```python
from build123d import *

# Parameters (mm, degrees)
SKETCH_1_W          = 55
SKETCH_1_H          = 60
EXTRUDE_1_DEPTH     = 3
SKETCH_2_W          = 30
SKETCH_2_H          = 22
EXTRUDE_2_DEPTH     = 3
SKETCH_3_R          = 1.05
CUT_EXTRUDE_1_DEPTH = 3
SKETCH_4_R          = 1.525
CUT_EXTRUDE_2_DEPTH = 3
SKETCH_5_R          = 1.5
CUT_EXTRUDE_3_DEPTH = 10
SKETCH_6_R          = 1.5
CUT_EXTRUDE_4_DEPTH = 10
CUT_EXTRUDE_5_DEPTH = 10
FILLET_1_R          = 2
FILLET_2_R          = 2


with BuildPart() as part:
    # 草图1 → 凸台-拉伸1 (new body)
    with BuildSketch(Plane.XY):
        Rectangle(SKETCH_1_W, SKETCH_1_H)
    extrude(amount=EXTRUDE_1_DEPTH)

    # 草图2 → 凸台-拉伸2 (add)
    with BuildSketch(Plane(origin=(0, 0, 0), x_dir=(-1, 0, 0), z_dir=(0, 0, -1))):
        with Locations((0, 30)):
            Rectangle(SKETCH_2_W, SKETCH_2_H)
    extrude(amount=-EXTRUDE_2_DEPTH)

    # 草图3 → 切除-拉伸1 (cut)
    with BuildSketch(Plane(origin=(0, 0, 0), x_dir=(-1, 0, 0), z_dir=(0, 0, -1))):
        with Locations((-16.05, 30)):
            Circle(SKETCH_3_R)
        with Locations((16.05, 30)):
            Circle(SKETCH_3_R)
    extrude(amount=-CUT_EXTRUDE_1_DEPTH, mode=Mode.SUBTRACT)

    # 草图4 → 切除-拉伸2 (cut)
    with BuildSketch(Plane.XY.offset(3)):
        with Locations((-10, 38)):
            Circle(SKETCH_4_R)
        with Locations((10, 38)):
            Circle(SKETCH_4_R)
    extrude(amount=-CUT_EXTRUDE_2_DEPTH, mode=Mode.SUBTRACT)

    # 草图5 → 切除-拉伸3 (cut)
    with BuildSketch(Plane(origin=(0, 0, 0), x_dir=(-1, 0, 0), z_dir=(0, 0, -1))):
        with Locations((-18.5, -17.5)):
            Circle(SKETCH_5_R)
        with Locations((18.5, -17.5)):
            Circle(SKETCH_5_R)
    extrude(amount=-CUT_EXTRUDE_3_DEPTH, mode=Mode.SUBTRACT)

    # 草图6 → 切除-拉伸4 (cut)
    with BuildSketch(Plane.XY.offset(3)):
        with Locations((20, 15)):
            Circle(SKETCH_6_R)
        with Locations((-20, 15)):
            Circle(SKETCH_6_R)
    extrude(amount=-CUT_EXTRUDE_4_DEPTH, mode=Mode.SUBTRACT)

    # 草图7 → 切除-拉伸5 (cut)
    with BuildSketch(Plane.XY.offset(3)):
        Polygon((-15, 24), (15, 24), (15, -12.5), (13.5, -12.5), (13.5, -24), (-13.5, -24), (-13.5, -12.5), (-15, -12.5), align=None)
    extrude(amount=-CUT_EXTRUDE_5_DEPTH, mode=Mode.SUBTRACT)

    # 圆角1
    # the kernel refuses this fillet: 2 mm, written as the material it adds along each edge
    with BuildSketch(Plane(origin=(-15, 24, 3), x_dir=(0, -1, 0), z_dir=(0, 0, -1))) as fillet_1_piece_1:
        with BuildLine():
            CenterArc((FILLET_1_R, -FILLET_1_R), FILLET_1_R, 90, 90)
            Line((0, -FILLET_1_R), (-FILLET_1_R * 0.02, -FILLET_1_R))
            Line((-FILLET_1_R * 0.02, -FILLET_1_R), (-FILLET_1_R * 0.02, FILLET_1_R * 0.02))
            Line((-FILLET_1_R * 0.02, FILLET_1_R * 0.02), (FILLET_1_R, FILLET_1_R * 0.02))
            Line((FILLET_1_R, FILLET_1_R * 0.02), (FILLET_1_R, 0))
        make_face()
    extrude(amount=3)
    with BuildSketch(Plane(origin=(15, 24, 3), x_dir=(0, -1, 0), z_dir=(0, 0, -1)), Plane(origin=(-13.5, -24, 3), x_dir=(0, 1, 0), z_dir=(0, 0, -1)), Plane(origin=(13.5, -24, 3), x_dir=(-1, 0, 0), z_dir=(0, 0, -1))) as fillet_1_piece_2:
        with BuildLine():
            CenterArc((FILLET_1_R, FILLET_1_R), FILLET_1_R, 180, 90)
            Line((0, FILLET_1_R), (-FILLET_1_R * 0.02, FILLET_1_R))
            Line((-FILLET_1_R * 0.02, FILLET_1_R), (-FILLET_1_R * 0.02, -FILLET_1_R * 0.02))
            Line((-FILLET_1_R * 0.02, -FILLET_1_R * 0.02), (FILLET_1_R, -FILLET_1_R * 0.02))
            Line((FILLET_1_R, -FILLET_1_R * 0.02), (FILLET_1_R, 0))
        make_face()
    extrude(amount=3)
    with BuildSketch(Plane(origin=(15, -12.5, 3), x_dir=(-1, 0, 0), z_dir=(0, 0, -1))) as fillet_1_piece_3:
        with BuildLine():
            CenterArc((2, 1.936491673), FILLET_1_R, 180, 75.522487814)
            Line((0, 1.936491673), (-0.04, 1.936491673))
            Line((-0.04, 1.936491673), (-0.04, 0))
            Line((-0.04, 0), (0, -0.04))
            ThreePointArc((0, -0.04), (0.75, -0.04), (1.49, -0.038729833))
            Line((1.49, -0.038729833), (1.5, 0))
        make_face()
    extrude(amount=3)
    with BuildSketch(Plane(origin=(-15, -12.5, 3), x_dir=(0, 1, 0), z_dir=(0, 0, -1))) as fillet_1_piece_4:
        with BuildLine():
            CenterArc((1.936491673, 2), FILLET_1_R, 194.477512186, 75.522487814)
            Line((0, 1.5), (-0.038729833, 1.49))
            ThreePointArc((-0.038729833, 1.49), (-0.04, 0.75), (-0.04, 0))
            Line((-0.04, 0), (0, -0.04))
            Line((0, -0.04), (1.936491673, -0.04))
            Line((1.936491673, -0.04), (1.936491673, 0))
        make_face()
    extrude(amount=3)

    # 圆角2
    fillet_2_edges = [part.edges().sort_by_distance(p)[0] for p in [
        (13.5, -12.5, 1.5),
        (-13.5, -12.5, 1.5),
    ]]
    fillet(fillet_2_edges, radius=FILLET_2_R)


solid = part.part
```
CAD build for the part. Positions are in the model's coordinates, mm. A direction names the side the tool comes from. Coordinates: 2 decimals unless noted, no trailing zeros. Order: outer loops, then holes, each group sorted by start corner. A loop starts at its lowest first (then second) coordinate and runs counter-clockwise, first axis right, second up. Notation, with made-up numbers: (45, 61) - (71, 61) arc R15 cw to (71, 88) - close; hole circle Ø10 at (0, -31.5). An arc over 180 degrees is marked (long way). Answer in a Markdown table with one row per item.
1. Slice it at D-D, the plane z = 1.8. Give the number of separate pieces and of enclosed holes in the cut face, then the cut area to 3 significant figures.
Answer:
| item | result |
|---|---|
| separate pieces | 1 |
| enclosed holes | 7 |
| area | 2,180 mm² |
2. Flat gauge pins, fed straight in: P1, Ø0.9, axis at x = -22, z = 2, coming from the +Y side; P2, Ø0.9, axis at y = 38, z = 1, coming from the +X side. Where does each tip first touch, or does it go through?
Answer:
| item | result |
|---|---|
| P1 | y = 30 |
| P2 | x = 15 |
3. Pull direction X, two halves, no side cores. Call faces 5 (the face through (15, 35, 1)), 6 (the face through (-14.43, 23.4, 1.52)), 7 (the face through (19, 6, 3)): +X half, -X half, draft (parallel to the pull), parting line (faces both ways), or undercut.
Answer:
| item | result |
|---|---|
| face 5 | +X half |
| face 6 | undercut |
| face 7 | draft |
4. Slice it at A-A, the plane y = -17.5. List the corners of the cut face in (x, z), then the cut area to 3 significant figures.
Answer:
| item | result |
|---|---|
| outline | (-27.5, 0) - (-20, 0) - (-20, 3) - (-27.5, 3) - close; (-17, 0) - (-13.5, 0) - (-13.5, 3) - (-17, 3) - close; (13.5, 0) - (17, 0) - (17, 3) - (13.5, 3) - close; (20, 0) - (27.5, 0) - (27.5, 3) - (20, 3) - close |
| area | 66.0 mm² |
5. Slice it at C-C, the plane y = 12. List the corners of the cut face in (x, z), then the cut area to 3 significant figures.
Answer:
| item | result |
|---|---|
| outline | (-27.5, 0) - (-15, 0) - (-15, 3) - (-27.5, 3) - close; (15, 0) - (27.5, 0) - (27.5, 3) - (15, 3) - close |
| area | 75.0 mm² |
6. Slice it at B-B, the plane x = 0. List the corners of the cut face in (y, z), then the cut area to 3 significant figures.
Answer:
| item | result |
|---|---|
| outline | (-30, 0) - (-24, 0) - (-24, 3) - (-30, 3) - close; (24, 0) - (41, 0) - (41, 3) - (24, 3) - close |
| area | 69.0 mm² |
7. 3-axis set-ups, long thin cutter, end or side, ignore diameter. For faces 1 (the face through (-15, 35, 1)), 2 (the face through (14.4, 23.43, 1.52)), 3 (the face through (0, 41, 1)), 4 (the face through (22, 30, 1)): which of +Z, -Z, +X, -X, +Y, -Y reach the whole face in a straight line?
Answer:
| item | result |
|---|---|
| face 1 | +Z, -Z, -X, +Y |
| face 2 | +Z, -Z |
| face 3 | +Z, -Z, +X, -X, +Y |
| face 4 | +Z, -Z, +X, +Y |
8. Drill centre lines: L1, parallel to X at y = -20, z = 0.45; L2, parallel to Y at x = 8, z = 1.6; L3, parallel to X at y = 6.5, z = 0.4. Where is each one in solid material? Low to high. Write a range as from..to.
Answer:
| item | result |
|---|---|
| L1 | -27.5..-13.5, 13.5..27.5 |
| L2 | -30..-24, 24..41 |
| L3 | -27.5..-15, 15..27.5 |
